Model file for the job. Use its own axes, mm. Give positions to 0.01 mm unless a question says otherwise; leave off trailing zeros. Write each loop counter-clockwise with the first axis right and the second up, starting at its lowest first coordinate (ties: lowest second). Pieces come first, ordered by that corner, then holes.
Autodesk Inventor part; units mm, degrees
ref_plane "작업 평면1" through (0, 1.7, 0) normal (0, 1, 0) x (1, 0, 0)
ref_plane "YZ Plane" through (0, 0, 0) normal (1, 0, 0) x (0, 1, 0)
ref_plane "XZ Plane" through (0, 0, 0) normal (0, 1, 0) x (-1, 0, 0)
sketch "스케치1" plane through (0, 0, 0) normal (0, 1, 0) x (-1, 0, 0)
  line L0 (-32.5919, 13.5) -> (-13.5, 32.5919)
  line L1 (-13.5, 32.5919) -> (13.5, 32.5919)
  line L2 (13.5, 32.5919) -> (32.5919, 13.5)
  line L3 (32.5919, 13.5) -> (32.5919, -13.5)
  line L4 (32.5919, -13.5) -> (13.5, -32.5919)
  line L5 (13.5, -32.5919) -> (-13.5, -32.5919)
  line L6 (-13.5, -32.5919) -> (-32.5919, -13.5)
  line L7 (-32.5919, -13.5) -> (-32.5919, 13.5)
  line L8 (34.9919, 14.4941) -> (34.9919, -14.4941)
  line L9 (34.9919, -14.4941) -> (14.4941, -34.9919)
  line L10 (14.4941, -34.9919) -> (-14.4941, -34.9919)
  line L11 (-14.4941, -34.9919) -> (-34.9919, -14.4941)
  line L12 (-34.9919, -14.4941) -> (-34.9919, 14.4941)
  line L13 (-34.9919, 14.4941) -> (-14.4941, 34.9919)
  line L14 (-14.4941, 34.9919) -> (14.4941, 34.9919)
  line L15 (14.4941, 34.9919) -> (34.9919, 14.4941)
  point P0 (0, 0)
  point P1 (0, 0)
  point P2 (0, 0)
  dimension "d0" = 27
  dimension "d1" = 2.4
extrude "돌출1" add sketch "스케치1" along normal blind 3.4 contours L0 L1 L2 L3 L4 L5 L6 L7 | L8 L9 L10 L11 L12 L13 L14 L15
sketch "스케치3" plane through (0, 0, 0) normal (0, -1, 0) x (1, 0, 0)
  line L0 (-13.5, 32.5919) -> (13.5, 32.5919)
  line L1 (13.5, 32.5919) -> (32.5919, 13.5)
  line L2 (32.5919, 13.5) -> (32.5919, -13.5)
  line L3 (32.5919, -13.5) -> (13.5, -32.5919)
  line L4 (13.5, -32.5919) -> (-13.5, -32.5919)
  line L5 (-13.5, -32.5919) -> (-32.5919, -13.5)
  line L6 (-32.5919, -13.5) -> (-32.5919, 13.5)
  line L7 (-32.5919, 13.5) -> (-13.5, 32.5919)
  line L8 (-13.9971, 33.7919) -> (13.9971, 33.7919)
  line L9 (13.9971, 33.7919) -> (33.7919, 13.9971)
  line L10 (33.7919, 13.9971) -> (33.7919, -13.9971)
  line L11 (33.7919, -13.9971) -> (13.9971, -33.7919)
  line L12 (13.9971, -33.7919) -> (-13.9971, -33.7919)
  line L13 (-13.9971, -33.7919) -> (-33.7919, -13.9971)
  line L14 (-33.7919, -13.9971) -> (-33.7919, 13.9971)
  line L15 (-33.7919, 13.9971) -> (-13.9971, 33.7919)
  line L16 (-13.1686, 31.7919) -> (13.1686, 31.7919)
  line L17 (13.1686, 31.7919) -> (31.7919, 13.1686)
  line L18 (31.7919, 13.1686) -> (31.7919, -13.1686)
  line L19 (31.7919, -13.1686) -> (13.1686, -31.7919)
  line L20 (13.1686, -31.7919) -> (-13.1686, -31.7919)
  line L21 (-13.1686, -31.7919) -> (-31.7919, -13.1686)
  line L22 (-31.7919, -13.1686) -> (-31.7919, 13.1686)
  line L23 (-31.7919, 13.1686) -> (-13.1686, 31.7919)
  point P0 (0, 0)
  point P1 (0, 0)
  point P2 (0, 0)
  point P3 (0, 0)
  dimension "d8" = 27
  dimension "d9" = 1.2
  dimension "d19" = 0.8
extrude "돌출3" cut sketch "스케치3" against normal blind 1.2 contours L0 L1 L2 L3 L4 L5 L6 L7 | L8 L9 L10 L11 L12 L13 L14 L15
sketch "스케치4" plane through (0, 3.4, 0) normal (0, 1, 0) x (1, 0, 0)
  line L0 (12.6716, -30.5919) -> (-12.6716, -30.5919)
  line L1 (-12.6716, -30.5919) -> (-30.5919, -12.6716)
  line L2 (-30.5919, -12.6716) -> (-30.5919, 12.6716)
  line L3 (-30.5919, 12.6716) -> (-12.6716, 30.5919)
  line L4 (-12.6716, 30.5919) -> (12.6716, 30.5919)
  line L5 (12.6716, 30.5919) -> (30.5919, 12.6716)
  line L6 (30.5919, 12.6716) -> (30.5919, -12.6716)
  line L7 (30.5919, -12.6716) -> (12.6716, -30.5919)
  line L8 (-31.7919, -13.1686) -> (-31.7919, 13.1686)
  point P0 (0, 0)
  point P1 (0, 0)
  dimension "d21" = 1.2
extrude "돌출4" cut sketch "스케치4" against normal blind 5
ref_plane "작업 평면1" through (0, 1.7, 0) normal (0, 1, 0) x (1, 0, 0)
sketch "스케치6" plane through (0, 0, 0) normal (0, -1, 0) x (1, 0, 0)
  line L0 (30.5919, -12.6716) -> (12.6716, -30.5919)
  line L1 (12.6716, -30.5919) -> (-12.6716, -30.5919)
  line L2 (-12.6716, -30.5919) -> (-30.5919, -12.6716)
  line L3 (-30.5919, -12.6716) -> (-30.5919, 12.6716)
  line L4 (-30.5919, 12.6716) -> (-12.6716, 30.5919)
  line L5 (-12.6716, 30.5919) -> (12.6716, 30.5919)
  line L6 (12.6716, 30.5919) -> (30.5919, 12.6716)
  line L7 (30.5919, 12.6716) -> (30.5919, -12.6716)
  line L8 (31.7919, 13.1686) -> (13.1686, 31.7919)
  line L9 (13.1686, 31.7919) -> (-13.1686, 31.7919)
  line L10 (-13.1686, 31.7919) -> (-31.7919, 13.1686)
  line L11 (-31.7919, 13.1686) -> (-31.7919, -13.1686)
  line L12 (-31.7919, -13.1686) -> (-13.1686, -31.7919)
  line L13 (-13.1686, -31.7919) -> (13.1686, -31.7919)
  line L14 (13.1686, -31.7919) -> (31.7919, -13.1686)
  line L15 (31.7919, -13.1686) -> (31.7919, 13.1686)
  point P0 (0, 0)
extrude "돌출7" cut sketch "스케치6" against normal blind 0.6
mirror "미러2" about plane through (0, 1.7, 0) normal (0, 1, 0) of "돌출7", "돌출3"
properties part number "팔각형 OV-PAM 5패턴 링 - 틈 너비 수정"
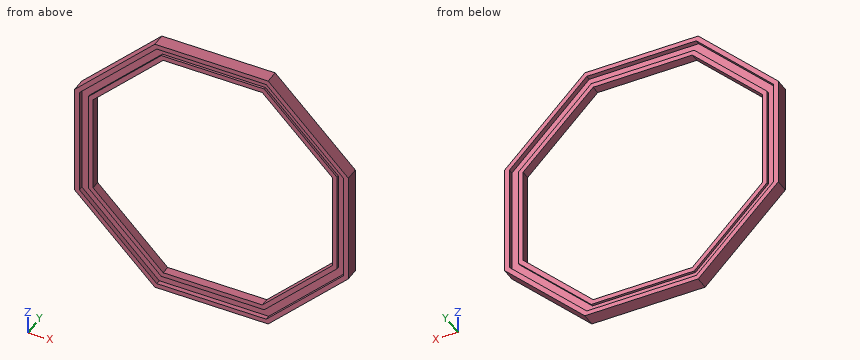
1. Slice it at B-B, the plane x = 1.5. Write the cut outline in (y, z), and give its area (3 significant figures).
Calculated:
outline: (0, -34.99) - (3.4, -34.99) - (3.4, -33.79) - (2.2, -33.79) - (2.2, -31.79) - (2.8, -31.79) - (2.8, -30.59) - (0.6, -30.59) - (0.6, -31.79) - (1.2, -31.79) - (1.2, -33.79) - (0, -33.79) - close; (0, 33.79) - (1.2, 33.79) - (1.2, 31.79) - (0.6, 31.79) - (0.6, 30.59) - (2.8, 30.59) - (2.8, 31.79) - (2.2, 31.79) - (2.2, 33.79) - (3.4, 33.79) - (3.4, 34.99) - (0, 34.99) - close
area: 17.4 mm2
2. Probe probe 1 along Z at (x, y) = (-5.5, 2.7); probe 2 along Z at (x, y) = (-24, 2.4). List the from-to ranges inside material, lowest first.
Calculated:
probe 1: z = -34.99 to -33.79, -31.79 to -30.59, 30.59 to 31.79, 33.79 to 34.99
probe 2: z = -25.49 to -23.79, -20.96 to -19.26, 19.26 to 20.96, 23.79 to 25.49
3. Slice it at A-A, the plane z = 2. Write the cut outline in (x, y).
Calculated:
outline: (-34.99, 0) - (-33.79, 0) - (-33.79, 1.2) - (-31.79, 1.2) - (-31.79, 0.6) - (-30.59, 0.6) - (-30.59, 2.8) - (-31.79, 2.8) - (-31.79, 2.2) - (-33.79, 2.2) - (-33.79, 3.4) - (-34.99, 3.4) - close; (30.59, 0.6) - (31.79, 0.6) - (31.79, 1.2) - (33.79, 1.2) - (33.79, 0) - (34.99, 0) - (34.99, 3.4) - (33.79, 3.4) - (33.79, 2.2) - (31.79, 2.2) - (31.79, 2.8) - (30.59, 2.8) - close
4. Pin check, flat tip, straight feed: P1, Ø10, axis at x = 13, z = 24, coming from the +Y side. Stop position of the tip, or through.
Calculated:
P1: stops at y = 2.8
